Model file for the job. Use its own axes, mm. Round coordinates to 2 decimals unless told otherwise and drop trailing zeros. Loops run counter-clockwise (first coordinate to the right, second up) from the corner with the lowest first, then second, coordinate; pieces in that order, holes last. Notation, with made-up numbers: (59, -37.75) - (63, -37.75) arc R31 cw to (63, 0.25) - close; hole circle Ø2 at (53.5, 27). An arc over 180 degrees is marked (long way). Use one line per item in the form item = value.
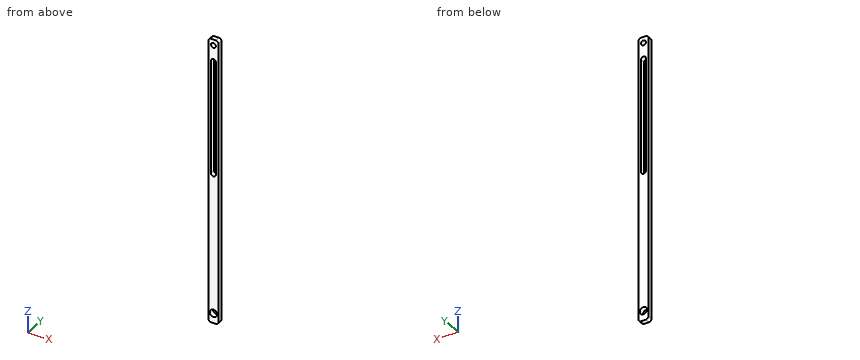
from build123d import *

# Parameters (mm, degrees)
F0_R     = 7.5
F0_R_2   = 5
F1_DEPTH = 10


with BuildPart() as f1:
    # F0 (on Front) → F1 (new body)
    with BuildSketch(Plane.XZ):
        with BuildLine():
            ThreePointArc((10, 285), (8.535534, 288.535534), (5, 290))
            Line((5, 290), (-5, 290))
            ThreePointArc((-5, 290), (-8.535534, 288.535534), (-10, 285))
            Line((-10, 285), (-10, -285))
            ThreePointArc((-10, -285), (-8.535534, -288.535534), (-5, -290))
            Line((-5, -290), (5, -290))
            ThreePointArc((5, -290), (8.535534, -288.535534), (10, -285))
            Line((10, -285), (10, 285))
        make_face()
        with Locations((0, -270)):
            Circle(F0_R, mode=Mode.SUBTRACT)
        with BuildLine():
            Line((5, 245), (5, 15))
            ThreePointArc((5, 15), (3.535534, 11.464466), (0, 10))
            ThreePointArc((0, 10), (-3.535534, 11.464466), (-5, 15))
            Line((-5, 15), (-5, 245))
            ThreePointArc((-5, 245), (-3.535534, 248.535534), (0, 250))
            ThreePointArc((0, 250), (3.535534, 248.535534), (5, 245))
        make_face(mode=Mode.SUBTRACT)
        with Locations((0, 278)):
            Circle(F0_R_2, mode=Mode.SUBTRACT)
    extrude(amount=F1_DEPTH)


solid = f1.part
1. Cut at A-A, the plane z = -270. Give the cut face in (x, y), plus the area to 3 significant figures.
Geometry check:
outline = (-10, -10) - (-7.5, -10) - (-7.5, 0) - (-10, 0) - close; (7.5, -10) - (10, -10) - (10, 0) - (7.5, 0) - close
area = 50.0 mm^2
2. Wall check: probe 1 along Z at (x, y) = (0, -2); probe 2 along X at (y, z) = (-4.75, -270); probe 3 along Z at (x, y) = (-1.5, -7.25). Give the ranges that are in metal, low to high.
Geometry check:
probe_1 = -290 to -277.5, -262.5 to 10, 250 to 273, 283 to 290
probe_2 = -10 to -7.5, 7.5 to 10
probe_3 = -290 to -277.35, -262.65 to 10.23, 249.77 to 273.23, 282.77 to 290
3. Cut at B-B, the plane y = -2.75. Give the cut face in (x, z).
Geometry check:
outline = (-10, -285) arc R5 ccw to (-5, -290) - (5, -290) arc R5 ccw to (10, -285) - (10, 285) arc R5 ccw to (5, 290) - (-5, 290) arc R5 ccw to (-10, 285) - close; hole circle Ø15 at (0, -270); hole (-5, 15) arc R5 ccw to (5, 15) - (5, 245) arc R5 ccw to (-5, 245) - close; hole circle Ø10 at (0, 278)
